from build123d import *

# Parameters (mm, degrees)
SKETCH_R          = 8.4
SKETCH_R_2        = 1.46
PAD_DEPTH         = 21.34
FILLET_R          = 0.5
SKETCH001_R       = 0.35
PAD001_DEPTH      = 10.67
PAD001_DEPTH_BACK = 3.5


with BuildPart() as fillet_body:
    # Sketch → Pad (new body)
    with BuildSketch(Plane.XY.offset(0.1)):
        with Locations((6.35, 0)):
            Circle(SKETCH_R)
        with Locations((6.35, 0)):
            Circle(SKETCH_R_2, mode=Mode.SUBTRACT)
    extrude(amount=PAD_DEPTH)

    # Fillet
    fillet_edges = [fillet_body.edges().sort_by_distance(p)[0] for p in [
        (4.89, 0, 21.44),
        (-2.05, 0, 21.44),
        (-2.05, 0, 0.1),
    ]]
    fillet(fillet_edges, radius=FILLET_R)


with BuildPart() as obj1:
    # Sketch001 → Pad001 (new body, two sides)
    with BuildSketch(Plane.XY.offset(0.5)) as pad001_sk:
        Circle(SKETCH001_R)
        with Locations((12.7, 0)):
            Circle(SKETCH001_R)
    extrude(amount=PAD001_DEPTH)
    extrude(pad001_sk.sketch, amount=-PAD001_DEPTH_BACK)

    # obj1: union Fillet body
    add(fillet_body.part)


solid = obj1.part
Verification items for the finished model (mm, model axes). Coordinates: 2 decimals unless noted, no trailing zeros. Loops run counter-clockwise (first coordinate to the right, second up) from the corner with the lowest first, then second, coordinate; pieces in that order, holes last. Notation, with made-up numbers: (-4, -7.5) -> (20, -7.5) arc R15 ccw to (20, -1.5) -> close; hole circle Ø1 at (28.5, 52.25). An arc over 180 degrees is marked (long way). Answer as a JSON object with one key per item and string values. Group by question number.
Item 1: Sectioned sample at A-A on x = 6.35. Record the boundary of the cut face in (y, z).
Item 2: Sectioned sample at B-B on y = 0. Record the boundary of the cut face in (x, z), plus the area to 3 significant figures.
Item 3: Mould release check, pull along Y, two halves, no side actions. Record for faces 1 (the cylindrical face through (4.89, 0.06, 10.37)), 2 (the flat face through (8, -2, 21.44)), 3 (the cylindrical face through (14.362, 2.523, 10.628)): +Y half, -Y half, draft (parallel to the pull), parting line (faces both ways), or undercut.
Item 4: Sectioned sample at C-C on z = 6.75. Record the boundary of the cut face in (x, y), plus the area to 3 significant figures.
Item 5: Depth check by flat-ended pin: pin 1 (4.5 mm diameter, centred on x = 5.5, y = -0.5, fed in from -Z); pin 2 (8 mm diameter, centred on y = 4.5, z = 17, fed in from +X); pin 3 (1.5 mm diameter, centred on x = 2.5, z = 2, fed in from -Y). Enter the tip coordinate at first touch or a pass-through.
Item 6: Scan lines: probe 1 along Y at (x, z) = (6.35, 10.75); probe 2 along Z at (x, y) = (6, -5.5); probe 3 along Y at (x, z) = (7, 4). Record each from-to range of solid material in increasing order.
Evaluation:
{
 "1": {"outline": "(-8.4, 0.6) arc R0.5 ccw to (-7.9, 0.1) -> (-1.46, 0.1) -> (-1.46, 20.94) arc R0.5 ccw to (-1.96, 21.44) -> (-7.9, 21.44) arc R0.5 ccw to (-8.4, 20.94) -> close; (1.46, 0.1) -> (7.9, 0.1) arc R0.5 ccw to (8.4, 0.6) -> (8.4, 20.94) arc R0.5 ccw to (7.9, 21.44) -> (1.96, 21.44) arc R0.5 ccw to (1.46, 20.94) -> close"},
 "2": {"outline": "(-2.05, 0.6) arc R0.5 ccw to (-1.55, 0.1) -> (-0.35, 0.1) -> (-0.35, -3) -> (0.35, -3) -> (0.35, 0.1) -> (4.89, 0.1) -> (4.89, 20.94) arc R0.5 ccw to (4.39, 21.44) -> (-1.55, 21.44) arc R0.5 ccw to (-2.05, 20.94) -> close; (7.81, 0.1) -> (12.35, 0.1) -> (12.35, -3) -> (13.05, -3) -> (13.05, 0.1) -> (14.25, 0.1) arc R0.5 ccw to (14.75, 0.6) -> (14.75, 20.94) arc R0.5 ccw to (14.25, 21.44) -> (8.31, 21.44) arc R0.5 ccw to (7.81, 20.94) -> close", "area": "300 mm²"},
 "3": {"face 1": "undercut", "face 2": "draft", "face 3": "parting line"},
 "4": {"outline": "circle Ø16.8 at (6.35, 0); hole circle Ø2.92 at (6.35, 0)", "area": "215 mm²"},
 "5": {"pin 1": "stops at z = 0.1", "pin 2": "stops at x = 14.74", "pin 3": "stops at y = -7.81"},
 "6": {"probe 1": "y = -8.4 to -1.46, 1.46 to 8.4", "probe 2": "z = 0.1 to 21.44", "probe 3": "y = -8.37 to -1.31, 1.31 to 8.37"}
}
